Autodesk Inventor part; units mm, degrees
ref_plane "Start plane" through (0, 0, 12.5) normal (0, 0, 1) x (1, 0, 0)
ref_plane "End plane" through (0, 0, 107.5) normal (0, 0, 1) x (1, 0, 0)
ref_plane "Work Plane4" through (0, 0, 12.5) normal (0, 0, -1) x (-1, 0, 0)
ref_plane "Start plane" through (0, 0, 12.5) normal (0, 0, 1) x (1, 0, 0)
ref_plane "End plane" through (0, 0, 107.5) normal (0, 0, 1) x (1, 0, 0)
sketch "Sketch" plane through (0, 0, 0) normal (0, 0, 1) x (1, 0, 0)
  line L0 (-12.5, -6.5) -> (-12.5, 6.5)
  line L1 (-6.5, 12.5) -> (6.5, 12.5)
  line L2 (12.5, 6.5) -> (12.5, -6.5)
  line L3 (6.5, -12.5) -> (-6.5, -12.5)
  arc A0 (-12.5, -6.5) -> (-6.5, -12.5) centre (-6.5, -6.5) ccw
  arc A1 (-6.5, 12.5) -> (-12.5, 6.5) centre (-6.5, 6.5) ccw
  arc A2 (12.5, 6.5) -> (6.5, 12.5) centre (6.5, 6.5) ccw
  arc A3 (6.5, -12.5) -> (12.5, -6.5) centre (6.5, -6.5) ccw
  arc A4 (-6.5, 9.5) -> (-9.5, 6.5) centre (-6.5, 6.5) ccw
  line L4 (-6.5, 9.5) -> (6.5, 9.5)
  arc A5 (9.5, 6.5) -> (6.5, 9.5) centre (6.5, 6.5) ccw
  line L5 (9.5, 6.5) -> (9.5, -6.5)
  arc A6 (6.5, -9.5) -> (9.5, -6.5) centre (6.5, -6.5) ccw
  line L6 (6.5, -9.5) -> (-6.5, -9.5)
  arc A7 (-9.5, -6.5) -> (-6.5, -9.5) centre (-6.5, -6.5) ccw
  line L7 (-9.5, -6.5) -> (-9.5, 6.5)
  line L8 (0, 19.2397) -> (0, -19.2397) construction
  line L9 (-19.2397, 0) -> (19.2397, 0) construction
  dimension "d7" = 6
  dimension "d10" = 25
  dimension "d11" = 25
  dimension "d12" = 3
  dimension "d15" = 12.5
  dimension "d16" = 12.5
extrude "Body" add sketch "Sketch" along normal up to surface (95 mm away) from surface at 12.5
sketch "Sketch3" plane through (0, 0, 0) normal (0, 0, 1) x (1, 0, 0)
  line L0 (0, 0) -> (10, 0)
ref_plane "Work Plane3" through (0, 0, 0) normal (0, -1, 0) x (1, 0, 0)
sketch "Sketch4" plane through (0, 0, 0) normal (0, -1, 0) x (1, 0, 0)
  line L0 (-2, 12.5) -> (12, 12.5)
  line L1 (-2, 107.5) -> (12, 107.5)
  dimension "d18" = 95
ref_plane "Work Plane4" through (0, 0, 12.5) normal (0, 0, -1) x (-1, 0, 0)
split "Split1" plane through (0, 0, 12.5) removes the side toward (0, 0, -1)
ref_plane "Work Plane5" through (0, -12.5, 107.5) normal (0, 0, 1) x (1, 0, 0)
split "Split2" plane through (0, -12.5, 107.5) removes the side toward (0, 0, 1)
equation "\"d7\" = G_IR"
equation "\"d10\" = G_H"
equation "\"d11\" = G_W"
equation "\"d12\" = G_T"
equation "\"d15\" = 0.5 * d10"
equation "\"d16\" = 0.5 * d11"
equation "\"d3\" = G_L"
equation "\"G_W\" = 25"
equation "\"G_H\" = 25"
equation "\"G_T\" = 3"
equation "\"G_IR\" = 6"
equation "\"G_L\" = d18"
equation "\"G_OFFSET_START\" = -12.5"
equation "\"G_OFFSET_END\" = -17.5"
equation "\"d13\" = -G_OFFSET_START"
equation "\"d14\" = G_OFFSET_END + B_L"
equation "\"B_L\" = 125"
properties part number "AS 1163 - C350L0 25x25x3.0 SHS - 95" material "Steel, Mild"
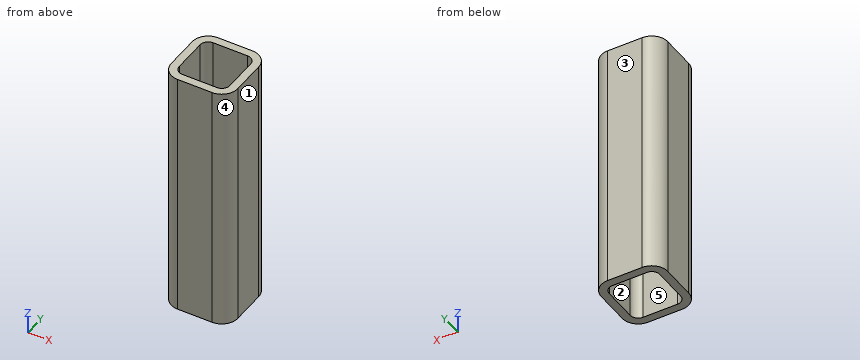
Could you check a few things on this model? Use its own coordinates, in mm. Face numbers are marked on the shaded views. A direction names the side the tool comes from. Give positions to 0.01 mm unless a question says otherwise; leave off trailing zeros. Order: outer loops, then holes, each group sorted by start corner. A loop starts at its lowest first (then second) coordinate and runs counter-clockwise, first axis right, second up.
Q1. Suppose I cut it at C-C, the plane z = 30. Write out the boundary of the cut face in (x, y), and give its area (3 significant figures).
Q2. Suppose I cut it at D-D, the plane x = 10.5. Write out the boundary of the cut face in (y, z).
Q3. If I drill on line 1 along X through (y, z) = (-6.75, 75); line 2 along Y through (x, z) = (4, 38); line 3 along X through (y, z) = (-8.75, 53), over which ranges is the centre line in solid material (lowest first)?
Q4. Suppose I cut it at A-A, the plane y = -3.25. Write out the boundary of the cut face in (x, z).
Q5. We'd pull the mould along Y, two halves only. Please class the marked faces 1, 2 and 3: +Y half, -Y half, draft (parallel to the pull), parting line (faces both ways), or undercut.
Q6. For the marked faces 4 and 5, which set-ups out of +Z, -Z, +X, -X, +Y, -Y let a thin tool reach every point of the face, with its end or its side?
Solution:
1. outline: (-12.5, -6.5) arc R6 ccw to (-6.5, -12.5) - (6.5, -12.5) arc R6 ccw to (12.5, -6.5) - (12.5, 6.5) arc R6 ccw to (6.5, 12.5) - (-6.5, 12.5) arc R6 ccw to (-12.5, 6.5) - close; hole (-9.5, -6.5) arc R3 ccw to (-6.5, -9.5) - (6.5, -9.5) arc R3 ccw to (9.5, -6.5) - (9.5, 6.5) arc R3 ccw to (6.5, 9.5) - (-6.5, 9.5) arc R3 ccw to (-9.5, 6.5) - close
1. area: 241 mm2
2. outline: (-10.97, 12.5) - (10.97, 12.5) - (10.97, 107.5) - (-10.97, 107.5) - close
3. line 1: x = -12.49 to -9.49, 9.49 to 12.49
3. line 2: y = -12.5 to -9.5, 9.5 to 12.5
3. line 3: x = -12.06 to -8.48, 8.48 to 12.06
4. outline: (-12.5, 12.5) - (-9.5, 12.5) - (-9.5, 107.5) - (-12.5, 107.5) - close; (9.5, 12.5) - (12.5, 12.5) - (12.5, 107.5) - (9.5, 107.5) - close
5. face 1: draft
5. face 2: undercut
5. face 3: +Y half
6. face 4: +Z, -Z, +X, -Y
6. face 5: +Z, -Z
